Job drawing, mm, ordinate dimensions from the low corner. One solid piece. A direction names the side the tool comes from. Give positions to 0.01 mm unless a question says otherwise; leave off trailing zeros. Write each loop counter-clockwise with the first axis right and the second up, starting at its lowest first coordinate (ties: lowest second). Pieces come first, ordered by that corner, then holes. Notation, with made-up numbers: M -33,88.25 L 3,88.25 A24 ccw 3,101.25 Z; hole C 5,10.5 d1. An arc over 180 degrees is marked long. Answer as CSV lines item,"result". Start each with the question number.
Item 1: 3-axis set-ups, long thin cutter, end or side, ignore diameter. For the marked faces 1, 2 and 3: which of +Z, -Z, +X, -X, +Y, -Y reach the whole face in a straight line?
Item 2: Band-saw the part on C-C, the plane y = 6.25. List the corners of the cut face in (x, z).
Item 3: Wall check: L1, parallel to X at y = 10.75, z = 1.5; L2, parallel to Z at x = 2, y = 27.5. Give the ranges that are in metal, low to high. Write a range as from..to.
Item 4: Band-saw the part on A-A, the plane z = 6.25. List the corners of the cut face in (x, y), then the cut area to 3 significant figures.
Item 5: Band-saw the part on D-D, the plane y = 13.75. List the corners of the cut face in (x, z).
Item 6: Band-saw the part on B-B, the plane x = 4. List the corners of the cut face in (y, z), then the cut area to 3 significant figures.
Item 7: Pin check, flat tips, straight feed: pin 1 (11 mm diameter, centred on x = 3, z = 25, fed in from +Y); pin 2 (1.5 mm diameter, centred on x = 22, y = 4, fed in from +Z); pin 3 (6 mm diameter, centred on y = 4, z = 25, fed in from +X); pin 4 (1 mm diameter, centred on x = 12.5, y = 11.5, fed in from -Z). Stop position of each tip, or through.
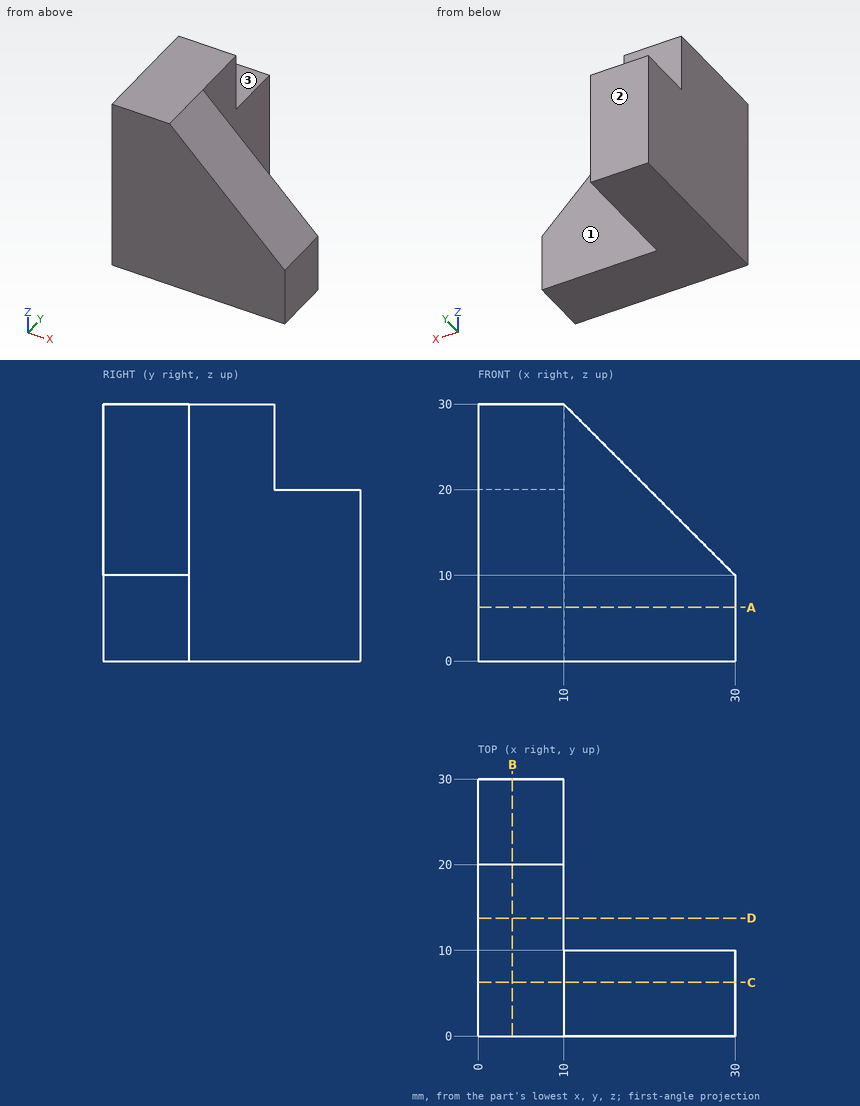
Output:
1,face 1,"+Z, -Z, +X, +Y"
1,face 2,"+Z, -Z, +X, -X, +Y"
1,face 3,"+Z, +X, -X, +Y"
2,outline,"M 0,0 L 30,0 L 30,10 L 10,30 L 0,30 Z"
3,L1,"0..10"
3,L2,"0..20"
4,outline,"M 0,0 L 30,0 L 30,10 L 10,10 L 10,30 L 0,30 Z"
4,area,"500 mm²"
5,outline,"M 0,0 L 10,0 L 10,30 L 0,30 Z"
6,outline,"M 0,0 L 30,0 L 30,20 L 20,20 L 20,30 L 0,30 Z"
6,area,"800 mm²"
7,pin 1,"y = 30"
7,pin 2,"z = 18.75"
7,pin 3,"x = 18"
7,pin 4,"through"
